from build123d import *

# Parameters (mm, degrees)
SKETCH1_R               = 3.96875
BOSS_EXTRUDE1_DEPTH     = 30
CUT_EXTRUDE1_DEPTH      = 31.520516921
CUT_EXTRUDE1_DEPTH_BACK = 31.520516921
CUT_EXTRUDE2_DEPTH      = 31.520516921
CUT_EXTRUDE2_DEPTH_BACK = 31.520516921


with BuildPart() as part:
    # Sketch1 → Boss-Extrude1 (new body)
    with BuildSketch(Plane.XY):
        Circle(SKETCH1_R)
    extrude(amount=BOSS_EXTRUDE1_DEPTH)

    # Sketch2 → Cut-Extrude1 (cut, two sides: drawn at the far end of the back side and taken through both)
    with BuildSketch(Plane(origin=(0, 0, 0), x_dir=(1, 0, 0), z_dir=(0, 1, 0)).offset(-CUT_EXTRUDE1_DEPTH_BACK)):
        with BuildLine():
            ThreePointArc((0, -30), (-2.806330038, -28.837580038), (-3.96875, -26.03125))
            Line((-3.96875, -26.03125), (-3.96875, -30))
            Line((-3.96875, -30), (0, -30))
        make_face()
        with BuildLine():
            Line((3.96875, -30), (3.96875, -26.03125))
            ThreePointArc((3.96875, -26.03125), (2.806330038, -28.837580038), (0, -30))
            Line((0, -30), (3.96875, -30))
        make_face()
    extrude(amount=CUT_EXTRUDE1_DEPTH + CUT_EXTRUDE1_DEPTH_BACK, mode=Mode.SUBTRACT)

    # Sketch3 → Cut-Extrude2 (cut, two sides: drawn at the far end of the back side and taken through both)
    with BuildSketch(Plane(origin=(0, 0, 0), x_dir=(1, 0, 0), z_dir=(0, 1, 0)).offset(-CUT_EXTRUDE2_DEPTH_BACK)):
        with BuildLine():
            ThreePointArc((0, 0), (2.806330038, -1.162419962), (3.96875, -3.96875))
            Line((3.96875, -3.96875), (3.96875, 0))
            Line((3.96875, 0), (0, 0))
        make_face()
        with BuildLine():
            Line((-3.96875, 0), (-3.96875, -3.96875))
            ThreePointArc((-3.96875, -3.96875), (-2.806330038, -1.162419962), (0, 0))
            Line((0, 0), (-3.96875, 0))
        make_face()
    extrude(amount=CUT_EXTRUDE2_DEPTH + CUT_EXTRUDE2_DEPTH_BACK, mode=Mode.SUBTRACT)


solid = part.part
Work out the finished part from the listing and answer in its coordinate system (mm). Round coordinates to 2 decimals unless told otherwise and drop trailing zeros. Order: outer loops, then holes, each group sorted by start corner. A loop starts at its lowest first (then second) coordinate and runs counter-clockwise, first axis right, second up. Notation, with made-up numbers: M 26.5,-39.5 L 85.5,-39.5 A23 ccw 85.5,-1.5 Z; hole C 33.5,64.5 d7. An arc over 180 degrees is marked long. One line per item, written item: value.
Q1. Flat-ended cylindrical pins translate along their axes: pin 1 (1 mm diameter, centred on x = 1.5, z = 20.5, fed in from -Y); pin 2 (2 mm diameter, centred on x = -2.5, y = -2, fed in from +Z); pin 3 (4 mm diameter, centred on x = 3, y = -1, fed in from -Z). Find the tip coordinate at first contact, or state that the pin passes through.
Derived:
pin 1: y = -3.84
pin 2: z = 29.71
pin 3: z = 0.13
Q2. Find section C-C on x = -3.5. Write down the section's boundary in (y, z), then the cut area to 3 significant figures.
Derived:
outline: M -1.87,2.1 L 1.87,2.1 L 1.87,27.9 L -1.87,27.9 Z
area: 96.6 mm²
Q3. Find section B-B on z = 20.5. Write down the section's boundary in (x, y).
Derived:
outline: C 0,0 d7.94
Q4. Straight lines are drawn through the part: line 1 (Z direction, x = 0.75, y = 3.75); line 2 (Y direction, x = -2.75, z = 27); line 3 (Y direction, x = -0.25, z = 10.5). For each, find the intervals that lie inside material, in ascending order.
Derived:
line 1: 0.07 to 29.93
line 2: -2.86 to 2.86
line 3: -3.96 to 3.96
Q5. Find section D-D on y = -3. Write down the section's boundary in (x, z).
Derived:
outline: M -2.6,0.97 A3.97 ccw 2.6,0.97 L 2.6,29.03 A3.97 ccw -2.6,29.03 Z
Q6. Find section A-A on y = 0. Write down the section's boundary in (x, z).
Derived:
outline: M -3.97,3.97 A3.97 ccw 3.97,3.97 L 3.97,26.03 A3.97 ccw -3.97,26.03 Z
